Build history of the part. All positions in model axes, mm. A direction names the side the tool comes from. Give positions to 0.01 mm unless a question says otherwise; leave off trailing zeros. Write each loop counter-clockwise with the first axis right and the second up, starting at its lowest first coordinate (ties: lowest second). Pieces come first, ordered by that corner, then holes. Notation, with made-up numbers: (37, 49.25) -> (49, 49.25) arc R21 ccw to (49, 70.25) -> close; hole circle Ø8 at (54, 81.25). An arc over 180 degrees is marked (long way). Write item = value, one per line. Start each with the question number.
Q1. Wall check: line 1 (X direction, y = 3.15, z = 0); line 2 (Y direction, x = 0.75, z = 2); line 3 (Y direction, x = -0.75, z = 3.5). Give the ranges that are in metal, low to high.
Q2. Mould opens along Z. For faces 3 (the face through (-2, 2, 0)), 4 (the face through (-1.7, 1.5, -0.5)), 5 (the face through (2.74, 1.01, -3.11)), 6 (the face through (-1.6, 1.5, 0.5)) say: pulls with the +Z half, pulls with the -Z half, needs draft (parallel to the pull), parting line crosses it, or undercut.
Q3. Saw through at A-A, the plane y = 1.4. List the corners of the cut face in (x, z), then the cut area to 3 significant figures.
Q4. Tool access for faces 1 (the face through (-1, 0, 0)), 2 (the face through (1.863, 1.507, -2.582)): list every direction of +Z, -Z, +X, -X, +Y, -Y with a clear straight run to the whole face (end or side of a thin tool).
Q5. Saw through at C-C, the plane y = 3.8. List the corners of the cut face in (x, z), then the cut area to 3 significant figures.
Q6. Saw through at B-B, the plane x = 0.25. List the corners of the cut face in (y, z).
Q7. Saw through at D-D, the plane z = -2.5. List the corners of the cut face in (x, y), then the cut area to 3 significant figures.
Q8. Drop flat-ended pins along their axis: P1, Ø3, axis at x = -4, z = 3, coming from the +Y side; P2, Ø2, axis at x = 0, z = -2, coming from the +Y side; P3, Ø0.8, axis at y = 1.5, z = 2, coming from the +X side. Give the stop position or say it passes through.
from build123d import *

# Parameters (mm, degrees)
SKETCH1_W           = 10.5
SKETCH1_H           = 8.3
BOSS_EXTRUDE1_DEPTH = 5
CUT_EXTRUDE1_DEPTH  = 10
SKETCH3_W           = 8.3
SKETCH3_H           = 5
BOSS_EXTRUDE2_DEPTH = 0.05
CUT_EXTRUDE2_DEPTH  = 3
SKETCH5_R           = 1.15
CUT_EXTRUDE3_DEPTH  = 5
CUT_EXTRUDE4_DEPTH  = 1
FILLET1_R           = 0.5


with BuildPart() as part:
    # Sketch1 → Boss-Extrude1 (new body)
    with BuildSketch(Plane(origin=(0, 0, 0), x_dir=(1, 0, 0), z_dir=(0, 1, 0))):
        Rectangle(SKETCH1_W, SKETCH1_H)
    extrude(amount=BOSS_EXTRUDE1_DEPTH)

    # Sketch2 → Cut-Extrude1 (cut)
    with BuildSketch(Plane(origin=(0, 5, 0), x_dir=(1, 0, 0), z_dir=(0, 1, 0))):
        with BuildLine():
            Line((1.75, 4.15), (3.75, 2.049390153))
            ThreePointArc((3.75, 2.049390153), (4.834935157, 1.26984251), (5.25, 0))
            Line((5.25, 0), (5.25, 4.15))
            Line((5.25, 4.15), (1.75, 4.15))
        make_face()
        with BuildLine():
            Line((3.75, -2.049390153), (1.75, -4.15))
            Line((1.75, -4.15), (3.75, -4.15))
            Line((3.75, -4.15), (5.25, -4.15))
            Line((5.25, -4.15), (5.25, 0))
            ThreePointArc((5.25, 0), (4.834935157, -1.26984251), (3.75, -2.049390153))
        make_face()
    extrude(amount=-CUT_EXTRUDE1_DEPTH, mode=Mode.SUBTRACT)

    # Sketch3 → Boss-Extrude2 (add)
    with BuildSketch(Plane.ZY.offset(5.25)):
        with Locations((0, 2.5)):
            Rectangle(SKETCH3_W, SKETCH3_H)
    extrude(amount=BOSS_EXTRUDE2_DEPTH)

    # Sketch4 → Cut-Extrude2 (cut)
    with BuildSketch(Plane(origin=(0, 5, 0), x_dir=(1, 0, 0), z_dir=(0, 1, 0))):
        with BuildLine():
            ThreePointArc((3.75, -2.049390153), (0.95, 0), (3.75, 2.049390153))
            Line((3.75, 2.049390153), (1.75, 4.15))
            Line((1.75, 4.15), (-5.3, 4.15))
            Line((-5.3, 4.15), (-5.3, -4.15))
            Line((-5.3, -4.15), (1.75, -4.15))
            Line((1.75, -4.15), (3.75, -2.049390153))
        make_face()
    extrude(amount=-CUT_EXTRUDE2_DEPTH, mode=Mode.SUBTRACT)

    # Sketch5 → Cut-Extrude3 (cut)
    with BuildSketch(Plane(origin=(0, 5, 0), x_dir=(1, 0, 0), z_dir=(0, 1, 0))):
        with Locations(Location((3.1, 0, 0), (0, 0, 270))):
            Circle(SKETCH5_R)
    extrude(amount=-CUT_EXTRUDE3_DEPTH, mode=Mode.SUBTRACT)

    # Sketch6 → Cut-Extrude4 (cut)
    with BuildSketch(Plane(origin=(0, 2, 0), x_dir=(1, 0, 0), z_dir=(0, 1, 0))):
        with BuildLine():
            Line((1.321758158, 3.15), (-4.3, 3.15))
            Line((-4.3, 3.15), (-4.3, 0.5))
            Line((-4.3, 0.5), (-1.21237994, 0.5))
            Line((-1.21237994, 0.5), (1.008947633, 0.5))
            ThreePointArc((1.008947633, 0.5), (1.503963979, 1.440544696), (2.389026153, 2.029043171))
            Line((2.389026153, 2.029043171), (1.321758158, 3.15))
        make_face()
        with BuildLine():
            Line((-1.21237994, -0.5), (-4.3, -0.5))
            Line((-4.3, -0.5), (-4.3, -3.15))
            Line((-4.3, -3.15), (1.321758158, -3.15))
            Line((1.321758158, -3.15), (2.389026153, -2.029043171))
            ThreePointArc((2.389026153, -2.029043171), (1.503963979, -1.440544696), (1.008947633, -0.5))
            Line((1.008947633, -0.5), (-1.21237994, -0.5))
        make_face()
    extrude(amount=-CUT_EXTRUDE4_DEPTH, mode=Mode.SUBTRACT)

    # Fillet1
    fillet1_edges = [part.edges().sort_by_distance(p)[0] for p in [
        (2.45, 5, 2.049390153),
    ]]
    fillet(fillet1_edges, radius=FILLET1_R)


solid = part.part
Report:
q1.line_1 = 0.95 to 1.95, 4.25 to 5.25
q1.line_2 = 0 to 1
q1.line_3 = 0 to 2
q2.face_3 = needs draft
q2.face_4 = undercut
q2.face_5 = pulls with the -Z half
q2.face_6 = undercut
q3.outline = (-5.3, -4.15) -> (1.75, -4.15) -> (3.75, -2.05) arc R2.15 ccw to (3.75, 2.05) -> (1.75, 4.15) -> (-5.3, 4.15) -> close; hole (-4.3, -3.15) -> (1.32, -3.15) -> (2.39, -2.03) arc R2.15 cw to (1.01, -0.5) -> (-4.3, -0.5) -> close; hole (-4.3, 0.5) -> (1.01, 0.5) arc R2.15 cw to (2.39, 2.03) -> (1.32, 3.15) -> (-4.3, 3.15) -> close; hole circle Ø2.3 at (3.1, 0)
q3.area = 39.9 mm2
q4.face_1 = +Z, -Z, +X, -X, -Y
q4.face_2 = +Y
q5.outline = circle Ø4.3 at (3.1, 0); hole circle Ø2.3 at (3.1, 0)
q5.area = 10.4 mm2
q6.outline = (0, -4.15) -> (2, -4.15) -> (2, -3.15) -> (1, -3.15) -> (1, -0.5) -> (2, -0.5) -> (2, 0.5) -> (1, 0.5) -> (1, 3.15) -> (2, 3.15) -> (2, 4.15) -> (0, 4.15) -> close
q7.outline = (-5.3, 0) -> (3.32, 0) -> (3.32, 2) -> (1.94, 2) -> (1.94, 1) -> (-4.3, 1) -> (-4.3, 2) -> (-5.3, 2) -> close
q7.area = 11.0 mm2
q8.P1 = 2
q8.P2 = 1
q8.P3 = 4.54
